from build123d import *

# Parameters (mm, degrees)
BOSS_EXTRUDE1_DEPTH = 0.25
BOSS_EXTRUDE2_DEPTH = 0.05


with BuildPart() as part:
    # Sketch1 → Boss-Extrude1 (new, symmetric)
    with BuildSketch(Plane(origin=(0, 0, 0), x_dir=(1, 0, 0), z_dir=(0, 1, 0))):
        Polygon((-5.877852523, -8.090169944), (5.877852523, -8.090169944), (9.510565163, 3.090169944), (0, 10), (-9.510565163, 3.090169944), align=None)
        Polygon((-5.667560078, -7.442956348), (-8.960012395, 2.690169944), (-3.63271264, -1.180339887), align=None, mode=Mode.SUBTRACT)
        Polygon((5.327299755, -7.690169944), (-5.327299755, -7.690169944), (0, -3.819660113), align=None, mode=Mode.SUBTRACT)
        Polygon((8.960012395, 2.690169944), (5.667560078, -7.442956348), (3.63271264, -1.180339887), align=None, mode=Mode.SUBTRACT)
        Polygon((-8.830044516, 3.090169944), (-0.210292445, 9.352786405), (-2.245139883, 3.090169944), align=None, mode=Mode.SUBTRACT)
        Polygon((0.210292445, 9.352786405), (8.830044516, 3.090169944), (2.245139883, 3.090169944), align=None, mode=Mode.SUBTRACT)
    extrude(amount=BOSS_EXTRUDE1_DEPTH, both=True)

    # Sketch2 → Boss-Extrude2 (add, symmetric)
    with BuildSketch(Plane(origin=(0, 0.25, 0), x_dir=(1, 0, 0), z_dir=(0, 1, 0))):
        Polygon((-2.245139883, 3.090169944), (-8.830044516, 3.090169944), (-0.210292445, 9.352786405), align=None)
        Polygon((-8.960012395, 2.690169944), (-3.63271264, -1.180339887), (-5.667560078, -7.442956348), align=None)
        Polygon((-5.327299755, -7.690169944), (0, -3.819660113), (5.327299755, -7.690169944), align=None)
        Polygon((8.960012395, 2.690169944), (5.667560078, -7.442956348), (3.63271264, -1.180339887), align=None)
        Polygon((8.830044516, 3.090169944), (2.245139883, 3.090169944), (0.210292445, 9.352786405), align=None)
    extrude(amount=BOSS_EXTRUDE2_DEPTH, both=True)


solid = part.part
CAD build for the part. Positions are in the model's coordinates, mm. Round coordinates to 2 decimals unless told otherwise and drop trailing zeros. Loops run counter-clockwise (first coordinate to the right, second up) from the corner with the lowest first, then second, coordinate; pieces in that order, holes last. Notation, with made-up numbers: M 37,76.5 L 42,76.5 A11 ccw 42,87.5 Z; hole C 56.5,27.25 d2. An arc over 180 degrees is marked long. One line per question, with ' | ' between items. Start each with the question number.
Item 1: Two-plate mould, pull along X, no slides. Class faces 1 (the flat face through (-3, 0, 6)), 2 (the flat face through (7.67, 0, 2.58)): pulls with the +X half, pulls with the -X half, needs draft (parallel to the pull), parting line crosses it, or undercut.
Item 2: Cut at B-B, the plane x = -1.75. Write the cut outline in (y, z), plus the area to 3 significant figures.
Item 3: Cut at C-C, the plane z = -5.75. Write the cut outline in (x, y), plus the area to 3 significant figures.
Item 4: Wall check: line 1 (X direction, y = -0.05, z = -1.75); line 2 (X direction, y = 0, z = 7); line 3 (X direction, y = -0.1, z = 4.5). Give the ranges that are in metal, low to high.
Item 5: Cut at A-A, the plane y = -0.1. Write the cut outline in (x, z).
Responses:
1) face 1: undercut | face 2: pulls with the +X half
2) outline: M -0.25,-8.73 L 0.25,-8.73 L 0.25,-8.23 L 0.3,-8.23 L 0.3,-4.61 L 0.25,-4.61 L 0.25,5.09 L 0.3,5.09 L 0.3,7.69 L 0.25,7.69 L 0.25,8.09 L -0.25,8.09 L -0.25,7.69 L 0.2,7.69 L 0.2,5.09 L -0.25,5.09 L -0.25,-4.61 L 0.2,-4.61 L 0.2,-8.23 L -0.25,-8.23 Z | area: 5.92 mm²
3) outline: M -5.85,-0.25 L -5.17,-0.25 L -5.17,0.2 L -1.38,0.2 L -1.38,-0.25 L 1.38,-0.25 L 1.38,0.2 L 5.17,0.2 L 5.17,-0.25 L 5.85,-0.25 L 5.85,0.25 L 5.17,0.25 L 5.17,0.3 L 1.38,0.3 L 1.38,0.25 L -1.38,0.25 L -1.38,0.3 L -5.17,0.3 L -5.17,0.25 L -5.85,0.25 Z | area: 2.82 mm²
4) line 1: x = -9.08 to -8.65, -7.67 to 7.67, 8.65 to 9.08 | line 2: x = -6.23 to -5.81, -5.52 to -4.38, 4.38 to 5.52, 5.81 to 6.23 | line 3: x = -7.04 to -6.62, -4.71 to -0.94, 0.94 to 4.71, 6.62 to 7.04
5) outline: M -9.51,-3.09 L 0,-10 L 9.51,-3.09 L 5.88,8.09 L -5.88,8.09 Z; hole M -8.96,-2.69 L -3.63,1.18 L -5.67,7.44 Z; hole M -8.83,-3.09 L -0.21,-9.35 L -2.25,-3.09 Z; hole M -5.33,7.69 L 0,3.82 L 5.33,7.69 Z; hole M 0.21,-9.35 L 8.83,-3.09 L 2.25,-3.09 Z; hole M 3.63,1.18 L 8.96,-2.69 L 5.67,7.44 Z
